from build123d import *

# Parameters (mm, degrees)
BOSS_EXTRUDE1_DEPTH = 10
BOSS_EXTRUDE3_DEPTH = 65
SKETCH3_W           = 6.566984135
SKETCH3_H           = 1.360389693
CUT_EXTRUDE2_DEPTH  = 65
BOSS_EXTRUDE4_DEPTH = 3.25
BOSS_EXTRUDE5_DEPTH = 2.25
SKETCH7_W           = 10
SKETCH7_H           = 5
BOSS_EXTRUDE6_DEPTH = 10
SKETCH8_R           = 2.5
CUT_EXTRUDE3_DEPTH  = 10
FILLET1_R           = 5
FILLET2_R           = 5
FILLET4_R           = 2.5
FILLET5_R           = 2.5
SKETCH9_W           = 100
SKETCH9_H           = 5.5
CUT_EXTRUDE4_DEPTH  = 100
BOSS_EXTRUDE7_DEPTH = 10
CUT_EXTRUDE5_DEPTH  = 150
SKETCH12_W          = 29.92089387
SKETCH12_H          = 33.203721342
CUT_EXTRUDE6_DEPTH  = 150
SKETCH14_W          = 19.184954217
SKETCH14_H          = 28.132637814
CUT_EXTRUDE7_DEPTH  = 150
SKETCH16_W          = 15.620456736
SKETCH16_H          = 10.822807293
CUT_EXTRUDE8_DEPTH  = 150
CUT_EXTRUDE9_DEPTH  = 10
CUT_EXTRUDE10_DEPTH = 10


with BuildPart() as part:
    # Sketch1 → Boss-Extrude1 (new body)
    with BuildSketch(Plane(origin=(0, 0, 0), x_dir=(1, 0, 0), z_dir=(0, 1, 0))):
        Polygon((-11.672910159, -34.563988547), (96.966700148, -34.563988547), (33.327089841, 29.07562176), (-11.672910159, 29.07562176), align=None)
    extrude(amount=BOSS_EXTRUDE1_DEPTH)

    # Sketch2 → Boss-Extrude3 (add)
    with BuildSketch(Plane.XY.offset(34.563988547)):
        Polygon((-11.672910159, 3.75), (-14.922910159, 3.75), (-14.922910159, 2), (-17.172910159, 2), (-17.172910159, 8), (-14.922910159, 8), (-14.922910159, 6.25), (-11.672910159, 6.25), align=None)
    extrude(amount=-BOSS_EXTRUDE3_DEPTH)

    # Sketch3 → Cut-Extrude2 (cut)
    with BuildSketch(Plane(origin=(0, 8, 0), x_dir=(1, 0, 0), z_dir=(0, 1, 0))):
        with Locations((-13.889418092, 29.755816607)):
            Rectangle(SKETCH3_W, SKETCH3_H)
    extrude(amount=-CUT_EXTRUDE2_DEPTH, mode=Mode.SUBTRACT)

    # Sketch4 → Boss-Extrude4 (add)
    with BuildSketch(Plane(origin=(0, 10, 0), x_dir=(1, 0, 0), z_dir=(0, 1, 0))):
        Polygon((91.663399289, -34.563988547), (28.023788982, 29.07562176), (25.520630977, 29.07562176), (89.160241283, -34.563988547), align=None)
    extrude(amount=BOSS_EXTRUDE4_DEPTH)

    # Sketch6 → Boss-Extrude5 (add)
    with BuildSketch(Plane(origin=(0, 13.25, 0), x_dir=(1, 0, 0), z_dir=(0, 1, 0))):
        Polygon((90.411820286, -34.563988547), (94.136820286, -34.563988547), (30.497209979, 29.07562176), (23.047209979, 29.07562176), (86.686820286, -34.563988547), align=None)
    extrude(amount=BOSS_EXTRUDE5_DEPTH)

    # Sketch7 → Boss-Extrude6 (add)
    with BuildSketch(Plane(origin=(0, 0, -29.07562176), x_dir=(-1, 0, 0), z_dir=(0, 0, -1))):
        with Locations((-28.327089841, 5)):
            Rectangle(SKETCH7_W, SKETCH7_H)
    extrude(amount=BOSS_EXTRUDE6_DEPTH)

    # Sketch8 → Cut-Extrude3 (cut)
    with BuildSketch(Plane(origin=(0, 7.5, 0), x_dir=(1, 0, 0), z_dir=(0, 1, 0))):
        with Locations(Location((28.327089841, 34.07562176, 0), (0, 0, 270))):
            Circle(SKETCH8_R)
    extrude(amount=-CUT_EXTRUDE3_DEPTH, mode=Mode.SUBTRACT)

    # Fillet1
    fillet1_edges = [part.edges().sort_by_distance(p)[0] for p in [
        (23.327089841, 5, -39.07562176),
    ]]
    fillet(fillet1_edges, radius=FILLET1_R)

    # Fillet2
    fillet2_edges = [part.edges().sort_by_distance(p)[0] for p in [
        (33.327089841, 5, -39.07562176),
    ]]
    fillet(fillet2_edges, radius=FILLET2_R - 0.0001)  # a hair under: the kernel refuses the full size

    # Fillet4
    fillet4_edges = [part.edges().sort_by_distance(p)[0] for p in [
        (23.327089841, 7.5, -31.57562176),
        (33.327089841, 7.5, -31.57567176),
        (24.791555935, 7.5, -37.611155666),
    ]]
    fillet(fillet4_edges, radius=FILLET4_R - 0.0001)  # a hair under: the kernel refuses the full size

    # Fillet5
    fillet5_edges = [part.edges().sort_by_distance(p)[0] for p in [
        (23.327089841, 2.5, -31.57562176),
        (33.327089841, 2.5, -31.57567176),
        (24.791555935, 2.5, -37.611155666),
        (31.862653036, 2.5, -37.611184955),
    ]]
    fillet(fillet5_edges, radius=FILLET5_R - 0.0001)  # a hair under: the kernel refuses the full size

    # Sketch9 → Cut-Extrude4 (cut)
    with BuildSketch(Plane.XY.offset(34.563988547)):
        with Locations((44.136820286, 12.75)):
            Rectangle(SKETCH9_W, SKETCH9_H)
    extrude(amount=-CUT_EXTRUDE4_DEPTH, mode=Mode.SUBTRACT)

    # Sketch10 → Boss-Extrude7 (add)
    with BuildSketch(Plane(origin=(0, 10, 0), x_dir=(1, 0, 0), z_dir=(0, 1, 0))):
        Polygon((96.966700148, -34.563988547), (89.895632336, -41.635056358), (7.416994707, 40.84358127), (14.488062519, 47.914649082), align=None)
    extrude(amount=BOSS_EXTRUDE7_DEPTH)

    # Sketch11 → Cut-Extrude5 (cut)
    with BuildSketch(Plane(origin=(65.765344347, 0, 65.765344347), x_dir=(0.7071067811865475, 0, -0.7071067811865477), z_dir=(0.7071067811865477, 0, 0.7071067811865475))):
        Polygon((40.542543722, 20), (40.542543722, 18), (42.592543722, 18), (42.592543722, 14), (35.492543722, 14), (35.492543722, 18), (37.542543722, 18), (37.542543722, 20), align=None)
    extrude(amount=-CUT_EXTRUDE5_DEPTH, mode=Mode.SUBTRACT)

    # Sketch12 → Cut-Extrude6 (cut)
    with BuildSketch(Plane(origin=(0, 10, 0), x_dir=(-1, 0, 0), z_dir=(0, -1, 0))):
        with Locations((-34.145401152, 45.677482431)):
            Rectangle(SKETCH12_W, SKETCH12_H)
    extrude(amount=-CUT_EXTRUDE6_DEPTH, mode=Mode.SUBTRACT)


with BuildPart() as cut_extrude6_piece_1:
    # of the separate pieces the step leaves, piece 1, a body of its own (cut_extrude6_pieces)
    add(part.part.solids().sort_by_distance((30.827189841, 2.5, -29.07562176))[0])

    # Sketch16 → Cut-Extrude8 (cut)
    with BuildSketch(Plane(origin=(0, 10, 0), x_dir=(-1, 0, 0), z_dir=(0, -1, 0))):
        with Locations((-90.634792892, -39.975392193)):
            Rectangle(SKETCH16_W, SKETCH16_H)
    extrude(amount=-CUT_EXTRUDE8_DEPTH, mode=Mode.SUBTRACT)

    # Sketch17 → Cut-Extrude9 (cut)
    with BuildSketch(Plane(origin=(0, 20, 0), x_dir=(1, 0, 0), z_dir=(0, 1, 0))):
        Polygon((92.966700148, -30.563988547), (78.824564524, -30.563988547), (73.824564524, -25.563988547), (87.966700148, -25.563988547), align=None)
    extrude(amount=-CUT_EXTRUDE9_DEPTH, mode=Mode.SUBTRACT)

    # Sketch18 → Cut-Extrude10 (cut)
    with BuildSketch(Plane(origin=(0, 10, 0), x_dir=(1, 0, 0), z_dir=(0, 1, 0))):
        with BuildLine():
            Line((27.059004739, 14.493613639), (16.811162643, 4.245771544))
            ThreePointArc((16.811162643, 4.245771544), (12.674223335, 4.245771544), (12.674223335, 8.382710852))
            Line((12.674223335, 8.382710852), (22.92206543, 18.630552948))
            ThreePointArc((22.92206543, 18.630552948), (27.059004739, 18.630552948), (27.059004739, 14.493613639))
        make_face()
        with BuildLine():
            Line((14.742692989, 3.517272066), (-5.595455146, 3.517272066))
            ThreePointArc((-5.595455146, 3.517272066), (-8.392424278, 6.314241198), (-5.595455146, 9.11121033))
            Line((-5.595455146, 9.11121033), (14.742692989, 9.11121033))
            ThreePointArc((14.742692989, 9.11121033), (17.539662121, 6.314241198), (14.742692989, 3.517272066))
        make_face()
    extrude(amount=-CUT_EXTRUDE10_DEPTH, mode=Mode.SUBTRACT)


with BuildPart() as cut_extrude6_piece_2:
    # of the separate pieces the step leaves, piece 2, a body of its own (cut_extrude6_pieces)
    add(part.part.solids().sort_by_distance((7.416994707, 10, -40.84358127))[0])

    # Sketch14 → Cut-Extrude7 (cut)
    with BuildSketch(Plane(origin=(0, 10, 0), x_dir=(-1, 0, 0), z_dir=(0, -1, 0))):
        with Locations((-9.592477109, 43.141940667)):
            Rectangle(SKETCH14_W, SKETCH14_H)
    extrude(amount=-CUT_EXTRUDE7_DEPTH, mode=Mode.SUBTRACT)


solid = cut_extrude6_piece_1.part
Model file for the job. Use its own axes, mm. A direction names the side the tool comes from. Give positions to 0.01 mm unless a question says otherwise; leave off trailing zeros. Loops run counter-clockwise (first coordinate to the right, second up) from the corner with the lowest first, then second, coordinate; pieces in that order, holes last.
Item 1: Slice it at C-C (x = 71). Write the cut outline in (y, z), plus the area to 3 significant figures.
Check values:
outline: (0, 8.6) - (20, 8.6) - (20, 13.66) - (18, 13.66) - (18, 10.77) - (14, 10.77) - (14, 20.81) - (18, 20.81) - (18, 17.91) - (20, 17.91) - (20, 22.74) - (10, 22.74) - (10, 34.56) - (0, 34.56) - close
area: 352 mm2
Item 2: Mould opens along X. For faces 5 (the face through (54, 14, -1)), 6 (the face through (58, 20, -2)), 7 (the face through (18.096, 5.07, -13.804)), 8 (the face through (32.575, 3.213, -31.541)) say: +X half, -X half, draft (parallel to the pull), parting line (faces both ways), or undercut.
Check values:
face 5: undercut
face 6: draft
face 7: undercut
face 8: +X half
Item 3: Slice it at A-A (x = 5). Write the cut outline in (y, z).
Check values:
outline: (0, -29.08) - (10, -29.08) - (10, -9.11) - (0, -9.11) - close; (0, -3.52) - (10, -3.52) - (10, 34.56) - (0, 34.56) - close
Item 4: Slice it at B-B (z = 23.5). Write the cut outline in (x, y), plus the area to 3 significant figures.
Check values:
outline: (-17.17, 2) - (-14.92, 2) - (-14.92, 3.75) - (-11.67, 3.75) - (-11.67, 0) - (85.9, 0) - (85.9, 20) - (80.84, 20) - (80.84, 18) - (83.73, 18) - (83.73, 14) - (73.69, 14) - (73.69, 18) - (76.59, 18) - (76.59, 20) - (71.76, 20) - (71.76, 10) - (-11.67, 10) - (-11.67, 6.25) - (-14.92, 6.25) - (-14.92, 8) - (-17.17, 8) - close
area: 1,090 mm2
Item 5: Which spindle directions (+Z, -Z, +X, -X, +Y, -Y) get a long thin tool onto all of the face, cutting with end or side? Do faces 1 (the face through (-16, 8, 3)), 2 (the face through (86, 13, 30.564)), 3 (the face through (51.72, 18.986, -1.373)), 4 (the face through (88, 14, 33)). Say none if no direction does.
Check values:
face 1: +Z, -Z, -X, +Y
face 2: +X, -X, +Y
face 3: +Y
face 4: none
Item 6: Slice it at D-D (z = -23). Write the cut outline in (x, y), plus the area to 3 significant figures.
Check values:
outline: (-17.17, 2) - (-14.92, 2) - (-14.92, 3.75) - (-11.67, 3.75) - (-11.67, 0) - (39.4, 0) - (39.4, 20) - (34.34, 20) - (34.34, 18) - (37.23, 18) - (37.23, 14) - (27.19, 14) - (27.19, 18) - (30.09, 18) - (30.09, 20) - (25.26, 20) - (25.26, 10) - (-11.67, 10) - (-11.67, 6.25) - (-14.92, 6.25) - (-14.92, 8) - (-17.17, 8) - close
area: 625 mm2
Item 7: Drill centre lines: line 1 along Z through (x, y) = (-3, 6.75); line 2 along Y through (x, z) = (16, -29); line 3 along Y through (x, z) = (91, 32). Where is each one in solid material? Low to high.
Check values:
line 1: z = -29.08 to -9.11, -3.52 to 34.56
line 2: y = 0 to 10
line 3: y = 0 to 14, 18 to 20
Item 8: Drop flat-ended pins along their axis: P1, Ø6, axis at x = 18.5, y = 5.5, coming from the -Z side; P2, Ø2.5, axis at x = 27, z = -34.5, coming from the +Y side; P3, Ø2.5, axis at x = -15.5, z = 3, coming from the -Y side. Give the stop position or say it passes through.
Check values:
P1: stops at z = -29.08
P2: stops at y = 7.5
P3: stops at y = 2
